from build123d import *

# Parameters (mm, degrees)
SALIENTE_EXTRUIR1_DEPTH = 190
CROQUIS2_R              = 3
CORTAR_EXTRUIR1_DEPTH   = 192.180542943
CORTAR_EXTRUIR3_DEPTH   = 192.180542943
CROQUIS4_W              = 33.127581221
CROQUIS4_H              = 30
CORTAR_EXTRUIR4_DEPTH   = 38
CROQUIS5_W              = 25
CROQUIS5_H              = 30
CORTAR_EXTRUIR5_DEPTH   = 30


with BuildPart() as part:
    # Croquis1 → Saliente-Extruir1 (new body)
    with BuildSketch(Plane.XY):
        with BuildLine():
            Line((-14, 15), (14, 15))
            ThreePointArc((14, 15), (14.707106781, 14.707106781), (15, 14))
            Line((15, 14), (15, -14))
            ThreePointArc((15, -14), (14.707106781, -14.707106781), (14, -15))
            Line((14, -15), (-14, -15))
            ThreePointArc((-14, -15), (-14.707106781, -14.707106781), (-15, -14))
            Line((-15, -14), (-15, 14))
            ThreePointArc((-15, 14), (-14.707106781, 14.707106781), (-14, 15))
        make_face()
    extrude(amount=-SALIENTE_EXTRUIR1_DEPTH)

    # Croquis2 → Cortar-Extruir1 (cut, through all)
    with BuildSketch(Plane.XY):
        Circle(CROQUIS2_R)
    extrude(amount=-CORTAR_EXTRUIR1_DEPTH, mode=Mode.SUBTRACT)

    # Croquis3 → Cortar-Extruir3 (cut, through all)
    with BuildSketch(Plane.XY):
        with BuildLine():
            Line((-5.492893219, 4.078679656), (-11.292893219, 9.878679656))
            ThreePointArc((-11.292893219, 9.878679656), (-12.382683432, 10.095452408), (-13, 9.171572875))
            Line((-13, 9.171572875), (-13, 5))
            ThreePointArc((-13, 5), (-14, 4), (-15, 5))
            Line((-15, 5), (-15, -5))
            ThreePointArc((-15, -5), (-14, -4), (-13, -5))
            Line((-13, -5), (-13, -9.171572875))
            ThreePointArc((-13, -9.171572875), (-12.382683432, -10.095452408), (-11.292893219, -9.878679656))
            Line((-11.292893219, -9.878679656), (-5.492893219, -4.078679656))
            ThreePointArc((-5.492893219, -4.078679656), (-5.276120467, -3.754256308), (-5.2, -3.371572875))
            Line((-5.2, -3.371572875), (-5.2, 3.371572875))
            ThreePointArc((-5.2, 3.371572875), (-5.276120467, 3.754256308), (-5.492893219, 4.078679656))
        make_face()
        with BuildLine():
            ThreePointArc((-9.171572875, 13), (-10.095452408, 12.382683432), (-9.878679656, 11.292893219))
            Line((-9.878679656, 11.292893219), (-4.078679656, 5.492893219))
            ThreePointArc((-4.078679656, 5.492893219), (-3.754256308, 5.276120467), (-3.371572875, 5.2))
            Line((-3.371572875, 5.2), (3.371572875, 5.2))
            ThreePointArc((3.371572875, 5.2), (3.754256308, 5.276120467), (4.078679656, 5.492893219))
            Line((4.078679656, 5.492893219), (9.878679656, 11.292893219))
            ThreePointArc((9.878679656, 11.292893219), (10.095452408, 12.382683432), (9.171572875, 13))
            Line((9.171572875, 13), (5, 13))
            ThreePointArc((5, 13), (4, 14), (5, 15))
            Line((5, 15), (-5, 15))
            ThreePointArc((-5, 15), (-4.292893219, 14.707106781), (-4, 14))
            ThreePointArc((-4, 14), (-4.292893219, 13.292893219), (-5, 13))
            Line((-5, 13), (-9.171572875, 13))
        make_face()
        with BuildLine():
            Line((9.878679656, -11.292893219), (4.078679656, -5.492893219))
            ThreePointArc((4.078679656, -5.492893219), (3.754256308, -5.276120467), (3.371572875, -5.2))
            Line((3.371572875, -5.2), (-3.371572875, -5.2))
            ThreePointArc((-3.371572875, -5.2), (-3.754256308, -5.276120467), (-4.078679656, -5.492893219))
            Line((-4.078679656, -5.492893219), (-9.878679656, -11.292893219))
            ThreePointArc((-9.878679656, -11.292893219), (-10.095452408, -12.382683432), (-9.171572875, -13))
            Line((-9.171572875, -13), (-5, -13))
            ThreePointArc((-5, -13), (-4.292893219, -13.292893219), (-4, -14))
            ThreePointArc((-4, -14), (-4.292893219, -14.707106781), (-5, -15))
            Line((-5, -15), (5, -15))
            ThreePointArc((5, -15), (4, -14), (5, -13))
            Line((5, -13), (9.171572875, -13))
            ThreePointArc((9.171572875, -13), (10.095452408, -12.382683432), (9.878679656, -11.292893219))
        make_face()
        with BuildLine():
            ThreePointArc((13, 9.171572875), (12.382683432, 10.095452408), (11.292893219, 9.878679656))
            Line((11.292893219, 9.878679656), (5.492893219, 4.078679656))
            ThreePointArc((5.492893219, 4.078679656), (5.276120467, 3.754256308), (5.2, 3.371572875))
            Line((5.2, 3.371572875), (5.2, -3.371572875))
            ThreePointArc((5.2, -3.371572875), (5.276120467, -3.754256308), (5.492893219, -4.078679656))
            Line((5.492893219, -4.078679656), (11.292893219, -9.878679656))
            ThreePointArc((11.292893219, -9.878679656), (12.382683432, -10.095452408), (13, -9.171572875))
            Line((13, -9.171572875), (13, -5))
            ThreePointArc((13, -5), (14, -4), (15, -5))
            Line((15, -5), (15, 5))
            ThreePointArc((15, 5), (14, 4), (13, 5))
            Line((13, 5), (13, 9.171572875))
        make_face()
    extrude(amount=-CORTAR_EXTRUIR3_DEPTH, mode=Mode.SUBTRACT)

    # Croquis4 → Cortar-Extruir4 (cut)
    with BuildSketch(Plane(origin=(0, 15, 0), x_dir=(1, 0, 0), z_dir=(0, 1, 0))):
        with Locations((-1.56379061, 15)):
            Rectangle(CROQUIS4_W, CROQUIS4_H)
    extrude(amount=-CORTAR_EXTRUIR4_DEPTH, mode=Mode.SUBTRACT)

    # Croquis5 → Cortar-Extruir5 (cut)
    with BuildSketch(Plane(origin=(15, 0, 0), x_dir=(0, 0, -1), z_dir=(1, 0, 0))):
        with Locations((42.5, 0)):
            Rectangle(CROQUIS5_W, CROQUIS5_H)
    extrude(amount=-CORTAR_EXTRUIR5_DEPTH, mode=Mode.SUBTRACT)


solid = part.part
Input: part model. Units: mm. Frame: model coordinates. A direction names the side the tool comes from. Give positions to 0.01 mm unless a question says otherwise; leave off trailing zeros. Loops run counter-clockwise (first coordinate to the right, second up) from the corner with the lowest first, then second, coordinate; pieces in that order, holes last. Notation, with made-up numbers: (-34.5, 32.25) -> (-16.5, 32.25) arc R27 ccw to (-16.5, 67.25) -> close; hole circle Ø10 at (-28.5, -30). An arc over 180 degrees is marked (long way). Answer as a JSON object with one key per item and string values. Group by question number.
Item 1: Cut plane A-A, the plane y = 0. Return the cut outline in (x, z), and give its area (3 significant figures).
Item 2: Line query: probe 1 along X at (y, z) = (-5.5, -134); probe 2 along X at (y, z) = (5.75, -146); probe 3 along Y at (x, z) = (0, -119). Output: solid intervals per line, ascending.
Item 3: Reachability of faces 1 (the flat face through (4, 0, -55)), 2 (the flat face through (0, 5.2, -122)), 3 (the flat face through (7, 13, -122)), 4 (the flat face through (5.2, 0, -122)) from +Z, -Z, +X, -X, +Y, -Y: full face, straight path, thin tool, end or side. Return the list, or none.
Item 4: Pin query (flat end, axial travel): P1, Ø6, axis at y = 0, z = -79, coming from the +X side; P2, Ø7.5, axis at x = 1, z = -149.5, coming from the -Y side; P3, Ø2, axis at y = -1, z = -122.5, coming from the -X side. Return the tip coordinate at first contact, or that it passes through.
Item 5: Pull-direction query (Y, two-part tool) for faces 5 (the flat face through (-15, 9, -122)), 6 (the flat face through (-6.938, -8.352, -121.555)), 7 (the flat face through (-10, 15, -122)); classes: released by +Y, released by -Y, zero draft, split by the parting line, or undercut.
Checks:
{
 "1": {"outline": "(-5.2, -190) -> (-3, -190) -> (-3, -55) -> (-5.2, -55) -> close; (3, -190) -> (5.2, -190) -> (5.2, -55) -> (3, -55) -> close", "area": "594 mm²"},
 "2": {"probe 1": "x = -15 to -13, -6.91 to -4.09, 4.09 to 6.91, 13 to 15", "probe 2": "x = -15 to -13, -7.16 to -4.34, 4.34 to 7.16, 13 to 15", "probe 3": "y = -5.2 to -3, 3 to 5.2"},
 "3": {"face 1": "+Z, +X, -X, +Y, -Y", "face 2": "+Z, -Z, +Y", "face 3": "+Z, -Z", "face 4": "+Z, -Z, +X"},
 "4": {"P1": "stops at x = 5.2", "P2": "stops at y = -14.97", "P3": "stops at x = -5.2"},
 "5": {"face 5": "zero draft", "face 6": "undercut", "face 7": "released by +Y"}
}
